from build123d import *

# Parameters (mm, degrees)
SKETCH1_W           = 40.5
SKETCH1_H           = 36
BOSS_EXTRUDE1_DEPTH = 10
SKETCH2_W           = 55.7
SKETCH2_H           = 2.5
BOSS_EXTRUDE2_DEPTH = 20
SKETCH3_R           = 4.4
BOSS_EXTRUDE3_DEPTH = 8
SKETCH4_W           = 45
SKETCH4_H           = 8.8
BOSS_EXTRUDE4_DEPTH = 2
SKETCH5_R           = 2.25
CUT_EXTRUDE1_DEPTH  = 2.5


with BuildPart() as part:
    # Sketch1 → Boss-Extrude1 (new, symmetric)
    with BuildSketch(Plane.XY):
        Rectangle(SKETCH1_W, SKETCH1_H)
    extrude(amount=BOSS_EXTRUDE1_DEPTH, both=True)

    # Sketch2 → Boss-Extrude2 (add)
    with BuildSketch(Plane.XY.offset(10)):
        with Locations((0, 9.75)):
            Rectangle(SKETCH2_W, SKETCH2_H)
    extrude(amount=-BOSS_EXTRUDE2_DEPTH)

    # Sketch3 → Boss-Extrude3 (add)
    with BuildSketch(Plane(origin=(0, 18, 0), x_dir=(1, 0, 0), z_dir=(0, 1, 0))):
        with Locations(Location((-9.25, 0, 0), (0, 0, 90))):
            Circle(SKETCH3_R)
    extrude(amount=BOSS_EXTRUDE3_DEPTH)

    # Sketch4 → Boss-Extrude4 (add)
    with BuildSketch(Plane(origin=(0, 26, 0), x_dir=(1, 0, 0), z_dir=(0, 1, 0))):
        with Locations((-9.25, 0)):
            Rectangle(SKETCH4_W, SKETCH4_H)
    extrude(amount=-BOSS_EXTRUDE4_DEPTH)

    # Sketch5 → Cut-Extrude1 (cut)
    with BuildSketch(Plane.XZ.offset(-8.5)):
        with Locations(Location((-24.05, -5.05, 0), (0, 0, 270))):
            Circle(SKETCH5_R)
        with Locations(Location((-24.05, 5.05, 0), (0, 0, 270))):
            Circle(SKETCH5_R)
        with Locations(Location((24.05, -5.05, 0), (0, 0, 270))):
            Circle(SKETCH5_R)
        with Locations(Location((24.05, 5.05, 0), (0, 0, 270))):
            Circle(SKETCH5_R)
    extrude(amount=-CUT_EXTRUDE1_DEPTH, mode=Mode.SUBTRACT)


solid = part.part
Source: CAD feature listing. Evaluate the final solid. Frame: model axes, mm. A direction names the side the tool comes from. Round coordinates to 2 decimals unless told otherwise and drop trailing zeros. Loops run counter-clockwise (first coordinate to the right, second up) from the corner with the lowest first, then second, coordinate; pieces in that order, holes last. Notation, with made-up numbers: (19, 78.25) -> (35, 78.25) arc R26 cw to (35, 98.25) -> close; hole circle Ø11 at (77, 78.5). An arc over 180 degrees is marked (long way). Answer as a JSON object with one key per item and string values. Group by question number.
Q1. Section query A-A (x = 6.5). Output: boundary loops of the cut face in (y, z), plus the area to 3 significant figures.
Q2. Contact query for flat-ended pins moving along their axis: P1, Ø7.5, axis at y = 16, z = 4.5, coming from the +X side; P2, Ø3.5, axis at x = 24.05, z = -5.05, coming from the -Y side (3 decimals); P3, Ø10, axis at y = 9.5, z = 7, coming from the -X side; P4, Ø8.5, axis at x = -25, z = 0.5, coming from the -Y side. Output: stop coordinate, or through.
Q3. Access query for faces 1 (the flat face through (13.25, 25, 0)), 2 (the flat face through (-20.25, -5, 0)), 3 (the flat face through (24, 8.5, 0)). Directions: +Z, -Z, +X, -X, +Y, -Y. A direction counts if a zero-diameter tool reaches every point of the face in a straight line with its end or side. Return the directions, or none.
Q4. Ray query, line 1 (X direction, y = 9.6, z = 5.05); line 2 (Y direction, x = -16, z = 0); line 3 (Z direction, x = -23, y = 24.5). Return the intervals inside material, ascending. Write a range as from..to.
Q5. Section query C-C (x = -24.05). Output: boundary loops of the cut face in (y, z).
Q6. Section query D-D (z = 0). Output: boundary loops of the cut face in (x, y), plus the area to 3 significant figures.
Q7. Mould query, pull axis Y, two halves, no side actions, for faces 4 (the flat face through (24, 11, 0)), 5 (the cylindrical face through (-26.046, 9.732, 4.012)), 6 (the flat face through (0, 18, 0)), 7 (the flat face through (-24, 11, 0)). Classes: pulls with the +Y half, pulls with the -Y half, needs draft (parallel to the pull), parting line crosses it, or undercut.
Q8. Section query B-B (z = 5.05). Output: boundary loops of the cut face in (x, y).
Completed:
{
 "1": {"outline": "(-18, -10) -> (18, -10) -> (18, 10) -> (-18, 10) -> close; (24, -4.4) -> (26, -4.4) -> (26, 4.4) -> (24, 4.4) -> close", "area": "738 mm²"},
 "2": {"P1": "x = 20.25", "P2": "through", "P3": "x = -27.85", "P4": "y = 8.5"},
 "3": {"face 1": "+Z, -Z, +X, +Y", "face 2": "+Z, -Z, -X, -Y", "face 3": "+Z, -Z, +X, -Y"},
 "4": {"line 1": "-27.85..-26.3, -21.8..21.8, 26.3..27.85", "line 2": "-18..18, 24..26", "line 3": "-4.4..4.4"},
 "5": {"outline": "(8.5, -10) -> (11, -10) -> (11, -7.3) -> (8.5, -7.3) -> close; (8.5, -2.8) -> (11, -2.8) -> (11, 2.8) -> (8.5, 2.8) -> close; (8.5, 7.3) -> (11, 7.3) -> (11, 10) -> (8.5, 10) -> close; (24, -4.4) -> (26, -4.4) -> (26, 4.4) -> (24, 4.4) -> close"},
 "6": {"outline": "(-31.75, 24) -> (-13.65, 24) -> (-13.65, 18) -> (-20.25, 18) -> (-20.25, 11) -> (-27.85, 11) -> (-27.85, 8.5) -> (-20.25, 8.5) -> (-20.25, -18) -> (20.25, -18) -> (20.25, 8.5) -> (27.85, 8.5) -> (27.85, 11) -> (20.25, 11) -> (20.25, 18) -> (-4.85, 18) -> (-4.85, 24) -> (13.25, 24) -> (13.25, 26) -> (-31.75, 26) -> close", "area": "1,640 mm²"},
 "7": {"face 4": "pulls with the +Y half", "face 5": "needs draft", "face 6": "undercut", "face 7": "undercut"},
 "8": {"outline": "(-27.85, 8.5) -> (-26.3, 8.5) -> (-26.3, 11) -> (-27.85, 11) -> close; (-21.8, 8.5) -> (-20.25, 8.5) -> (-20.25, -18) -> (20.25, -18) -> (20.25, 8.5) -> (21.8, 8.5) -> (21.8, 11) -> (20.25, 11) -> (20.25, 18) -> (-20.25, 18) -> (-20.25, 11) -> (-21.8, 11) -> close; (26.3, 8.5) -> (27.85, 8.5) -> (27.85, 11) -> (26.3, 11) -> close"}
}
